from build123d import *

# Parameters (mm, degrees)
BASE_FLANGE1_START = -38.1
BASE_FLANGE1_DEPTH = 76.2
SKETCH6_R          = 26.162
SKETCH6_R_2        = 4.7879
CUT_EXTRUDE1_DEPTH = 94.544815593
SKETCH7_R          = 4.9657
CUT_EXTRUDE2_DEPTH = 90.4661943
FILLET1_R          = 15.875
FILLET2_R          = 3.175


# Read off the part's stored shape, not the designer's step: Base-Flange1
with BuildPart() as part:
    # Base-Flange1 outline → Base-Flange1 (new body)
    with BuildSketch(Plane(origin=(0, 0, 0), x_dir=(0, 0, -1), z_dir=(1, 0, 0)).offset(BASE_FLANGE1_START)):
        with BuildLine():
            Line((0, 56.830523199), (0, 0))
            Line((0, 0), (6.35, 0))
            Line((6.35, 0), (6.35, 56.830523199))
            ThreePointArc((6.35, 56.830523199), (6.924192259, 58.651628384), (8.439086045, 59.81404727))
            Line((8.439086045, 59.81404727), (37.974116762, 70.563919319))
            Line((37.974116762, 70.563919319), (35.802288852, 76.530967461))
            Line((35.802288852, 76.530967461), (6.267258135, 65.781095412))
            ThreePointArc((6.267258135, 65.781095412), (1.722576778, 62.293838755), (0, 56.830523199))
        make_face()
    extrude(amount=BASE_FLANGE1_DEPTH)

    # Sketch6 → Cut-Extrude1 (cut, through all)
    with BuildSketch(Plane.XY):
        Circle(SKETCH6_R)
        with Locations((0, 44.45)):
            Circle(SKETCH6_R_2)
    extrude(amount=-CUT_EXTRUDE1_DEPTH, mode=Mode.SUBTRACT)

    # Sketch7 → Cut-Extrude2 (cut, through all)
    with BuildSketch(Plane(origin=(0, 56.071911069, 20.408506608), x_dir=(1, 0, 0), z_dir=(0, 0.9396926207859093, 0.34202014332566627))):
        with Locations(Location((0, 43.943279101, 0), (0, 0, 270))):
            Circle(SKETCH7_R)
    extrude(amount=-CUT_EXTRUDE2_DEPTH, mode=Mode.SUBTRACT)

    # Fillet1
    fillet1_edges = [part.edges().sort_by_distance(p)[0] for p in [
        (38.1, 73.54744339, -36.888202807),
        (-38.1, 73.54744339, -36.888202807),
    ]]
    fillet(fillet1_edges, radius=FILLET1_R)

    # Fillet2
    fillet2_edges = [part.edges().sort_by_distance(p)[0] for p in [
        (26.162, 0, -3.175),
        (-26.162, 0, -3.175),
        (38.1, 0, -3.175),
        (-38.1, 0, -3.175),
    ]]
    fillet(fillet2_edges, radius=FILLET2_R)


solid = part.part
Geometry check sheet. Reference: the model listing, model coordinates, mm. A direction names the side the tool comes from. Round coordinates to 2 decimals unless told otherwise and drop trailing zeros. Loops run counter-clockwise (first coordinate to the right, second up) from the corner with the lowest first, then second, coordinate; pieces in that order, holes last.
Item 1: Access from +Z, -Z, +X, -X, +Y, -Y to the whole of each face (thin tool, end or side, straight path). Record for faces 4 (the cylindrical face through (27.021, 0.833, -3.219)), 5 (the flat face through (-1, 34, -6.35)), 6 (the cylindrical face through (37.19, 0.95, -3.22)).
Item 2: Cross-section at B-B on x = 1. Record the boundary of the cut face in (y, z) (3 decimals).
Item 3: Cross-section at C-C on z = -3. Record the boundary of the cut face in (x, y) (3 decimals).
Item 4: Cross-section at A-A on y = 44.45. Record the boundary of the cut face in (x, z).
Item 5: Mould release check, pull along Z, two halves, no side actions. Record for faces 1 (the cylindrical face through (-1.902, 66.591, -17.645)), 2 (the cylindrical face through (0.536, 26.157, -3.131)), 3 (the flat face through (-0.533, 68.842, -14.678)): pulls with the +Z half, pulls with the -Z half, needs draft (parallel to the pull), parting line crosses it, or undercut.
Item 6: Gauge pin test, flat ends, axial feed: pin 1 (8 mm diameter, centred on x = 12, z = -30, fed in from +Y) (3 decimals); pin 2 (1 mm diameter, centred on x = 17, z = -12, fed in from -Y); pin 3 (6 mm diameter, centred on x = -13.5, y = 42.5, fed in from -Z). Record the tip position at first contact, or that the pin passes through.
Item 7: Cross-section at D-D on x = -14. Record the boundary of the cut face in (y, z) (3 decimals).
Item 8: Thickness scan on line 1 (X direction, y = 44, z = -3); line 2 (Z direction, x = -23, y = 43); line 3 (X direction, y = 17.5, z = -5). Record the ranges inside material, lowest first.
Answer sheet:
1. face 4: +Z, -Z, -Y
1. face 5: -Z, +X, -X, -Y
1. face 6: +Z, -Z, +X, -Y
2. outline: (26.143, -6.35) - (39.768, -6.35) - (39.768, 0) - (26.143, 0) - close; (49.132, -6.35) - (56.831, -6.35) arc R3.175 cw to (59.814, -8.439) - (63.471, -18.486) - (69.438, -16.314) - (65.781, -6.267) arc R9.525 ccw to (56.831, 0) - (49.132, 0) - close; (66.798, -27.627) - (70.564, -37.974) - (76.531, -35.802) - (72.765, -25.455) - close
3. outline: (-38.1, 3.175) arc R3.175 ccw to (-34.925, 0) - (-29.165, 0) arc R3.175 ccw to (-26.008, 2.831) arc R26.162 cw to (26.008, 2.831) arc R3.175 ccw to (29.165, 0) - (34.925, 0) arc R3.175 ccw to (38.1, 3.175) - (38.1, 63.77) - (-38.1, 63.77) - close; hole circle Ø9.576 at (0, 44.45)
4. outline: (-38.1, -6.35) - (-4.79, -6.35) - (-4.79, 0) - (-38.1, 0) - close; (4.79, -6.35) - (38.1, -6.35) - (38.1, 0) - (4.79, 0) - close
5. face 1: undercut
5. face 2: needs draft
5. face 3: pulls with the +Z half
6. pin 1: stops at y = 75.875
6. pin 2: stops at y = 60.93
6. pin 3: stops at z = -6.35
7. outline: (22.101, -6.35) - (56.831, -6.35) arc R3.175 cw to (59.814, -8.439) - (70.564, -37.974) - (76.531, -35.802) - (65.781, -6.267) arc R9.525 ccw to (56.831, 0) - (22.101, 0) - close
8. line 1: x = -38.1 to -4.77, 4.77 to 38.1
8. line 2: z = -6.35 to 0
8. line 3: x = -38.1 to -19.45, 19.45 to 38.1
